Here's how the part is built. I have some questions about the finished solid (model axes, mm). Face numbers are marked on the shaded views. A direction names the side the tool comes from. Round coordinates to 2 decimals unless told otherwise and drop trailing zeros. Write each loop counter-clockwise with the first axis right and the second up, starting at its lowest first coordinate (ties: lowest second). Pieces come first, ordered by that corner, then holes. Notation, with made-up numbers: M 59,50 L 73,50 A16 cw 73,62 Z; hole C 30,-7 d5. An arc over 180 degrees is marked long. Use a Markdown table: item, result. Add a question column.
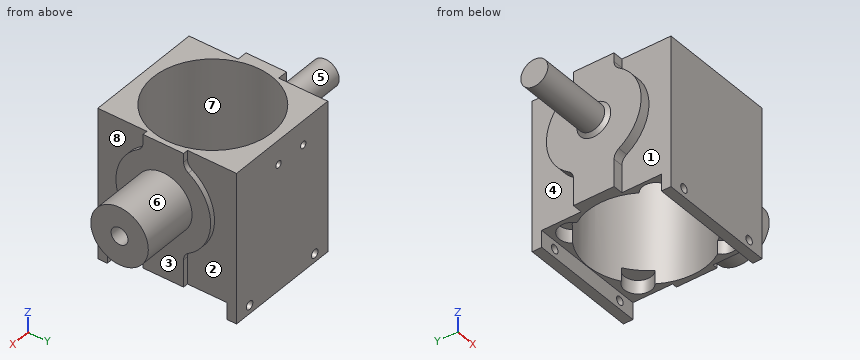
```python
from build123d import *

# Parameters (mm, degrees)
BOSS_EXTRUDE1_DEPTH             = 44.5
BOSS_EXTRUDE2_REACH             = 63.096
SKETCH3_R                       = 14
BOSS_EXTRUDE2_DIRECTION_2_REACH = 63.096
SKETCH5_R                       = 17.56
CUT_EXTRUDE2_DEPTH              = 54.110733378
SKETCH6_W                       = 5
SKETCH6_H                       = 35.4
CUT_EXTRUDE3_DEPTH              = 63.934489749
FILLET1_R                       = 3
SKETCH7_R                       = 8.5
BOSS_EXTRUDE4_DEPTH             = 16.78
SKETCH8_R                       = 4
BOSS_EXTRUDE5_DEPTH             = 22.8
CHAMFER1_SIZE                   = 1
M3X0_5_TAPPED_HOLE1_D           = 2.5
M2_5X0_45_TAPPED_HOLE1_REACH    = 76.405
M2_5X0_45_TAPPED_HOLE1_BORE_R   = 1.025
M6X1_0_TAPPED_HOLE1_D           = 5
M6X1_0_TAPPED_HOLE1_DEPTH       = 10
M6X1_0_TAPPED_HOLE1_TIP         = 1.502151548
SKETCH16_R                      = 4
CUT_EXTRUDE4_DEPTH              = 4


with BuildPart() as part:
    # Sketch1 → Boss-Extrude1 (new body)
    with BuildSketch(Plane.XY):
        Polygon((-17.5, 20.5), (17.5, 20.5), (17.5, 6), (19, 6), (19, -6), (17.5, -6), (17.5, -20.5), (-17.5, -20.5), (-17.5, -6), (-20.5, -6), (-20.5, 6), (-17.5, 6), align=None)
    extrude(amount=BOSS_EXTRUDE1_DEPTH)

    # Boss-Extrude2: up to this face of the body (flat: up to its plane)
    boss_extrude2_end = Plane(part.part.faces().sort_by_distance((-20.5, 0, 22.25))[0])
    # Sketch3 → Boss-Extrude2 (add, up to the picked face)
    with BuildSketch(Plane.ZY.offset(17.5), mode=Mode.PRIVATE) as boss_extrude2_sk1:
        with Locations((27.5, 0)):
            Circle(SKETCH3_R)
    boss_extrude2_tool1 = split(extrude(boss_extrude2_sk1.sketch, amount=BOSS_EXTRUDE2_REACH, mode=Mode.PRIVATE), bisect_by=boss_extrude2_end, keep=Keep.BOTH, mode=Mode.PRIVATE)
    add(boss_extrude2_tool1.solids().sort_by(Axis((-17.5, 0, 27.5), (-1, 0, 0)))[0])

    # Boss-Extrude2 direction 2: up to this face of the body (flat: up to its plane)
    boss_extrude2_direction_2_end = Plane(part.part.faces().sort_by_distance((19, 0, 22.25))[0])
    # Sketch3 → Boss-Extrude2 direction 2 (add, up to the picked face)
    with BuildSketch(Plane.ZY.offset(17.5), mode=Mode.PRIVATE) as boss_extrude2_direction_2_sk1:
        with Locations((27.5, 0)):
            Circle(SKETCH3_R)
    boss_extrude2_direction_2_tool1 = split(extrude(boss_extrude2_direction_2_sk1.sketch, amount=-BOSS_EXTRUDE2_DIRECTION_2_REACH, mode=Mode.PRIVATE), bisect_by=boss_extrude2_direction_2_end, keep=Keep.BOTH, mode=Mode.PRIVATE)
    add(boss_extrude2_direction_2_tool1.solids().sort_by(Axis((-17.5, 0, 27.5), (1, 0, 0)))[0])

    # Sketch5 → Cut-Extrude2 (cut, through all)
    with BuildSketch(Plane.XY.offset(44.5)):
        Circle(SKETCH5_R)
    extrude(amount=-CUT_EXTRUDE2_DEPTH, mode=Mode.SUBTRACT)

    # Sketch6 → Cut-Extrude3 (cut, through all)
    with BuildSketch(Plane.ZY.offset(20.5)):
        with Locations((2.5, 0)):
            Rectangle(SKETCH6_W, SKETCH6_H)
    extrude(amount=-CUT_EXTRUDE3_DEPTH, mode=Mode.SUBTRACT)

    # Fillet1
    fillet1_edges = [part.edges().sort_by_distance(p)[0] for p in [
        (18.25, -6, 40.149110641),
        (18.25, -6, 14.850889359),
        (18.25, 6, 14.850889359),
        (18.25, 6, 40.149110641),
        (-19, 6, 14.850889359),
        (-19, 6, 40.149110641),
        (-19, -6, 40.149110641),
        (-19, -6, 14.850889359),
    ]]
    fillet(fillet1_edges, radius=FILLET1_R)

    # Sketch7 → Boss-Extrude4 (add)
    with BuildSketch(Plane(origin=(19, 0, 0), x_dir=(0, 0, -1), z_dir=(1, 0, 0))):
        with Locations((-27.5, 0)):
            Circle(SKETCH7_R)
    extrude(amount=BOSS_EXTRUDE4_DEPTH)

    # Sketch8 → Boss-Extrude5 (add)
    with BuildSketch(Plane.ZY.offset(20.5)):
        with Locations((27.5, 0)):
            Circle(SKETCH8_R)
    extrude(amount=BOSS_EXTRUDE5_DEPTH)

    # Chamfer1
    chamfer1_edges = [part.edges().sort_by_distance(p)[0] for p in [
        (-20.5, 0, 23.5),
    ]]
    chamfer(chamfer1_edges, length=CHAMFER1_SIZE)

    # M3x0.5 Tapped Hole1 (through all)
    with Locations(Plane(origin=(0, -20.5, 0), x_dir=(-1, 0, 0), z_dir=(0, -1, 0))):
        with Locations((-12.5, -2.5), (12.5, -2.5)):
            Hole(M3X0_5_TAPPED_HOLE1_D / 2)

    # M2.5x0.45 Tapped Hole1 bore → M2.5x0.45 Tapped Hole1 (cut, up to next)
    with BuildSketch(Plane(origin=(0, 20.5, 0), x_dir=(1, 0, 0), z_dir=(0, 1, 0)), mode=Mode.PRIVATE) as m2_5x0_45_tapped_hole1_sk1:
        with Locations((-8.1, -37.35)):
            Circle(M2_5X0_45_TAPPED_HOLE1_BORE_R)
    m2_5x0_45_tapped_hole1_tool1 = extrude(m2_5x0_45_tapped_hole1_sk1.sketch, amount=-M2_5X0_45_TAPPED_HOLE1_REACH, mode=Mode.PRIVATE) & part.part
    # M2.5x0.45 Tapped Hole1 bore → M2.5x0.45 Tapped Hole1 (cut, up to next)
    with BuildSketch(Plane(origin=(0, 20.5, 0), x_dir=(1, 0, 0), z_dir=(0, 1, 0)), mode=Mode.PRIVATE) as m2_5x0_45_tapped_hole1_sk2:
        with Locations((1.4, -37.35)):
            Circle(M2_5X0_45_TAPPED_HOLE1_BORE_R)
    m2_5x0_45_tapped_hole1_tool2 = extrude(m2_5x0_45_tapped_hole1_sk2.sketch, amount=-M2_5X0_45_TAPPED_HOLE1_REACH, mode=Mode.PRIVATE) & part.part
    add(m2_5x0_45_tapped_hole1_tool1.solids().sort_by_distance((-8.1, 20.5, 37.35))[0], mode=Mode.SUBTRACT)
    add(m2_5x0_45_tapped_hole1_tool2.solids().sort_by_distance((1.4, 20.5, 37.35))[0], mode=Mode.SUBTRACT)

    # M6x1.0 Tapped Hole1
    with Locations(Plane(origin=(35.78, 0, 0), x_dir=(0, 0, -1), z_dir=(1, 0, 0))):
        with Locations((-27.5, 0)):
            Hole(M6X1_0_TAPPED_HOLE1_D / 2, depth=M6X1_0_TAPPED_HOLE1_DEPTH)
            with Locations((0, 0, -(M6X1_0_TAPPED_HOLE1_DEPTH + M6X1_0_TAPPED_HOLE1_TIP / 2))):  # 118° drill point
                Cone(0, M6X1_0_TAPPED_HOLE1_D / 2, M6X1_0_TAPPED_HOLE1_TIP, mode=Mode.SUBTRACT)

    # Sketch16 → Cut-Extrude4 (cut)
    with BuildSketch(Plane(origin=(0, 0, 5), x_dir=(-1, 0, 0), z_dir=(0, 0, -1))):
        with Locations((12.346045823, 12.48714349)):
            Circle(SKETCH16_R)
        with Locations((12.522297379, -12.310490175)):
            Circle(SKETCH16_R)
        with Locations((-12.275336286, -12.486741731)):
            Circle(SKETCH16_R)
        with Locations((-12.451587842, 12.310891934)):
            Circle(SKETCH16_R)
    extrude(amount=-CUT_EXTRUDE4_DEPTH, mode=Mode.SUBTRACT)


solid = part.part
```
Item 1: For pin 1 Ø0.9 at (x, z) = (-19.5, 9.5) entering from -Y; pin 2 Ø1.5 at (x, z) = (-19.5, 9) entering from +Y; pin 3 Ø3 at (x, y) = (-28, 4.5) entering from +Z, each with a flat end and sliding along its axis, tell me the tip position at first contact or that it passes through.
Item 2: Imagine slicing it at A-A on z = 2.5. List the corners of the cut face in (x, y) for me.
Item 3: On a 3-axis mill with a long thin cutter (end or side, diameter ignored), from which of +Z, -Z, +X, -X, +Y, -Y can I reach the whole of each face in a straight line? I mean the marked faces 1, 2, 3, 4 and 5. Say none if no direction works.
Item 4: Imagine slicing it at D-D on x = -8.1. List the corners of the cut face in (y, z) for me (3 decimals).
Item 5: Imagine slicing it at C-C on z = 37.35. List the corners of the cut face in (x, y) for me (3 decimals), plus the area to 3 significant figures.
Item 6: I need wall thicknesses on probe 1 along Z at (x, y) = (-12.5, 19.95); probe 2 along X at (y, z) = (0, 39); probe 3 along Z at (x, y) = (12.5, 15). Which ranges of each line are inside material? Lowest first, please. Write a range as from..to.
Item 7: If we mould it in two halves opening along Y, with no side actions, what happens to the marked faces 6, 7 and 8? For each: +Y half, -Y half, draft (parallel to the pull), parting line (faces both ways), or undercut.
Item 8: Imagine slicing it at B-B on y = 12.5. List the corners of the cut face in (x, z) for me, plus the area to 3 significant figures.
The answers:
| question | item | result |
|---|---|---|
| 1 | pin 1 | y = -6 |
| 1 | pin 2 | y = 6 |
| 1 | pin 3 | z = 30.15 |
| 2 | outline | M -17.5,-20.5 L -13.75,-20.5 L -13.75,-17.7 L -17.5,-17.7 Z; M -17.5,17.7 L -13.75,17.7 L -13.75,20.5 L -17.5,20.5 Z; M -11.25,-20.5 L 11.25,-20.5 L 11.25,-17.7 L -11.25,-17.7 Z; M -11.25,17.7 L 11.25,17.7 L 11.25,20.5 L -11.25,20.5 Z; M 13.75,-20.5 L 17.5,-20.5 L 17.5,-17.7 L 13.75,-17.7 Z; M 13.75,17.7 L 17.5,17.7 L 17.5,20.5 L 13.75,20.5 Z |
| 3 | face 1 | -X, -Y |
| 3 | face 2 | +X, +Y |
| 3 | face 3 | +X |
| 3 | face 4 | -X, +Y |
| 3 | face 5 | -X |
| 4 | outline | M -20.5,0 L -17.7,0 L -17.7,5 L -15.58,5 L -15.58,44.5 L -20.5,44.5 Z; M 15.58,5 L 17.7,5 L 17.7,0 L 20.5,0 L 20.5,36.325 L 15.58,36.325 Z; M 15.58,38.375 L 20.5,38.375 L 20.5,44.5 L 15.58,44.5 Z |
| 5 | outline | M -20.5,-9.949 L -17.5,-9.949 L -17.5,-20.5 L 17.5,-20.5 L 17.5,-9.949 L 19,-9.949 L 19,9.949 L 17.5,9.949 L 17.5,20.5 L 2.425,20.5 L 2.425,17.392 A17.56 cw long -9.125,15.003 L -9.125,20.5 L -17.5,20.5 L -17.5,9.949 L -20.5,9.949 Z; M -7.075,16.072 A17.56 cw 0.375,17.556 L 0.375,20.5 L -7.075,20.5 Z |
| 5 | area | 540 mm² |
| 6 | probe 1 | 0..1.25, 3.75..44.5 |
| 6 | probe 2 | -20.5..-17.56, 17.56..19 |
| 6 | probe 3 | 9..44.5 |
| 7 | face 6 | parting line |
| 7 | face 7 | undercut |
| 7 | face 8 | draft |
| 8 | outline | M -20.5,21.2 L -17.5,21.2 L -17.5,5 L -16.35,5 L -16.35,9 L -12.33,9 L -12.33,44.5 L -17.5,44.5 L -17.5,33.8 L -20.5,33.8 Z; M 12.33,9 L 16.45,9 L 16.45,5 L 17.5,5 L 17.5,21.2 L 19,21.2 L 19,33.8 L 17.5,33.8 L 17.5,44.5 L 12.33,44.5 Z |
| 8 | area | 432 mm² |
